Input: part model. Units: mm. Frame: model coordinates. Round coordinates to 2 decimals unless told otherwise and drop trailing zeros. Write each loop counter-clockwise with the first axis right and the second up, starting at its lowest first coordinate (ties: lowest second). Pieces come first, ordered by that corner, then holes. Notation, with made-up numbers: M 37,68 L 67,68 A22 cw 67,89 Z; hole C 80,67.25 d8. An arc over 180 degrees is marked long. Write each question's results on one line, items separated by ' | '. Start each with the question number.
```python
from build123d import *

# Parameters (mm, degrees)
BOSS_EXTRUDE1_DEPTH = 6
SKETCH2_W           = 20
SKETCH2_H           = 6
CUT_EXTRUDE1_DEPTH  = 7
LPATTERN1_COUNT     = 5
LPATTERN1_PITCH     = 40
SKETCH3_W           = 6
SKETCH3_H           = 20
CUT_EXTRUDE2_DEPTH  = 7
LPATTERN2_COUNT     = 5
LPATTERN2_PITCH     = 40
SKETCH4_W           = 6
SKETCH4_H           = 6
CUT_EXTRUDE3_DEPTH  = 10
SKETCH5_W           = 6
SKETCH5_H           = 20
CUT_EXTRUDE4_DEPTH  = 10
LPATTERN3_COUNT     = 2
LPATTERN3_PITCH     = 40
SKETCH7_W           = 6
SKETCH7_H           = 20
CUT_EXTRUDE5_DEPTH  = 10
LPATTERN4_COUNT     = 5
LPATTERN4_PITCH     = 40
SKETCH8_R           = 15
CUT_EXTRUDE6_DEPTH  = 10
SKETCH9_R           = 7.5
CUT_EXTRUDE7_DEPTH  = 7


with BuildPart() as part:
    # Sketch1 → Boss-Extrude1 (new body)
    with BuildSketch(Plane.XY):
        Polygon((-17.330934256, 199.427419355), (102.669065744, 199.427419355), (102.669065744, 53.427419355), (182.669065744, 53.427419355), (182.669065744, -6.572580645), (102.669065744, -6.572580645), (-17.330934256, -6.572580645), align=None)
    extrude(amount=BOSS_EXTRUDE1_DEPTH)

    # Sketch2 → Cut-Extrude1 (cut, through all)
    with BuildSketch(Plane.XY.offset(6)):
        with Locations((12.669065744, -3.572580645)):
            Rectangle(SKETCH2_W, SKETCH2_H)
    cut_extrude1 = extrude(amount=-CUT_EXTRUDE1_DEPTH, mode=Mode.SUBTRACT)

    # LPattern1: Cut-Extrude1 ×5
    with Locations(*[(i * LPATTERN1_PITCH, 0, 0) for i in range(1, LPATTERN1_COUNT)]):
        add(cut_extrude1, mode=Mode.SUBTRACT)

    # Sketch3 → Cut-Extrude2 (cut, through all)
    with BuildSketch(Plane.XY):
        with Locations((99.669065744, 23.427419355)):
            Rectangle(SKETCH3_W, SKETCH3_H)
    cut_extrude2 = extrude(amount=CUT_EXTRUDE2_DEPTH, mode=Mode.SUBTRACT)

    # LPattern2: Cut-Extrude2 ×5
    with Locations(*[(0, i * LPATTERN2_PITCH, 0) for i in range(1, LPATTERN2_COUNT)]):
        add(cut_extrude2, mode=Mode.SUBTRACT)

    # Sketch4 → Cut-Extrude3 (cut)
    with BuildSketch(Plane.XY.offset(6)):
        with Locations((99.669065744, 196.427419355)):
            Rectangle(SKETCH4_W, SKETCH4_H)
    extrude(amount=-CUT_EXTRUDE3_DEPTH, mode=Mode.SUBTRACT)

    # Sketch5 → Cut-Extrude4 (cut)
    with BuildSketch(Plane.XY.offset(6)):
        with Locations((179.669065744, 43.427419355)):
            Rectangle(SKETCH5_W, SKETCH5_H)
    cut_extrude4 = extrude(amount=-CUT_EXTRUDE4_DEPTH, mode=Mode.SUBTRACT)

    # LPattern3: Cut-Extrude4 ×2
    with Locations(*[(0, -i * LPATTERN3_PITCH, 0) for i in range(1, LPATTERN3_COUNT)]):
        add(cut_extrude4, mode=Mode.SUBTRACT)

    # Sketch7 → Cut-Extrude5 (cut)
    with BuildSketch(Plane.XY.offset(6)):
        with Locations((-14.330934256, 189.427419355)):
            Rectangle(SKETCH7_W, SKETCH7_H)
    cut_extrude5 = extrude(amount=-CUT_EXTRUDE5_DEPTH, mode=Mode.SUBTRACT)

    # LPattern4: Cut-Extrude5 ×5
    with Locations(*[(0, -i * LPATTERN4_PITCH, 0) for i in range(1, LPATTERN4_COUNT)]):
        add(cut_extrude5, mode=Mode.SUBTRACT)

    # Sketch8 → Cut-Extrude6 (cut)
    with BuildSketch(Plane(origin=(0, 0, 0), x_dir=(-1, 0, 0), z_dir=(0, 0, -1))):
        with Locations((-42.669065744, 43.427419355)):
            Circle(SKETCH8_R)
    extrude(amount=-CUT_EXTRUDE6_DEPTH, mode=Mode.SUBTRACT)

    # Sketch9 → Cut-Extrude7 (cut, through all)
    with BuildSketch(Plane(origin=(0, 0, 0), x_dir=(-1, 0, 0), z_dir=(0, 0, -1))):
        with Locations((-147.669065744, 18.427419355)):
            Circle(SKETCH9_R)
    extrude(amount=-CUT_EXTRUDE7_DEPTH, mode=Mode.SUBTRACT)


solid = part.part
```
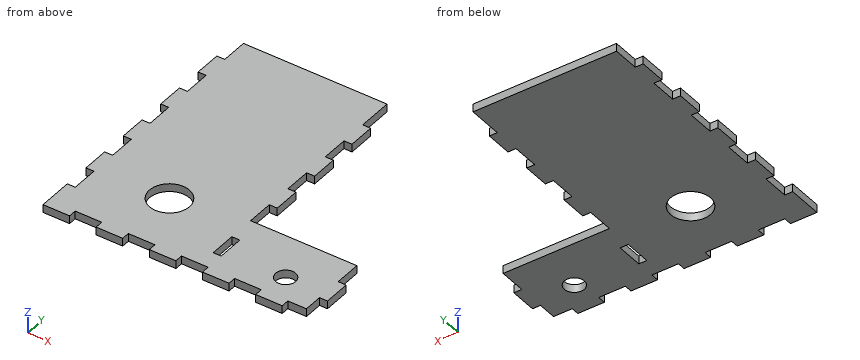
1. Cut plane B-B on y = 31. Output: boundary loops of the cut face in (x, z).
2. Contact query for flat-ended pins moving along their axis: P1, Ø1.8, axis at x = 168.5, z = 4, coming from the -Y side; P2, Ø1.8, axis at x = -13, z = 4.5, coming from the +Y side; P3, Ø1.8, axis at x = 100, z = 4, coming from the +Y side; P4, Ø12, axis at x = 147.67, y = 18.43, coming from the +Z side. Output: stop coordinate, or through.
3. Cut plane A-A on x = 33. Output: boundary loops of the cut face in (y, z).
4. Line query: L1, parallel to Y at x = 13.5, z = 0.4; L2, parallel to Y at x = 34, z = 1.55; L3, parallel to X at y = 73, z = 2.6. Output: solid intervals per line, ascending. Write a range as from..to.
5. Cut plane C-C on y = 64. Output: boundary loops of the cut face in (x, z).
6. Cut plane D-D on x = 85.5. Output: boundary loops of the cut face in (y, z).
Answers follow:
1) outline: M -11.33,0 L 34.27,0 L 34.27,6 L -11.33,6 Z; M 51.07,0 L 96.67,0 L 96.67,6 L 51.07,6 Z; M 102.67,0 L 182.67,0 L 182.67,6 L 102.67,6 Z
2) P1: stops at y = -0.57 | P2: stops at y = 179.43 | P3: stops at y = 173.43 | P4: passes through
3) outline: M -6.57,0 L 31.96,0 L 31.96,6 L -6.57,6 Z; M 54.9,0 L 199.43,0 L 199.43,6 L 54.9,6 Z
4) L1: y = -0.57..199.43 | L2: y = -6.57..31.19, 55.67..199.43 | L3: x = -11.33..96.67
5) outline: M -11.33,0 L 96.67,0 L 96.67,6 L -11.33,6 Z
6) outline: M -0.57,0 L 199.43,0 L 199.43,6 L -0.57,6 Z
